```python
from build123d import *

# Parameters (mm, degrees)
BOSS_EXTRUDE1_DEPTH      = 175
BOSS_EXTRUDE1_DEPTH_BACK = 175
SKETCH1_R                = 12.7
SKETCH2_R                = 12.7
BOSS_EXTRUDE2_DEPTH      = 15
BOSS_EXTRUDE3_START      = 15
SKETCH3_R                = 12.7
BOSS_EXTRUDE3_DEPTH      = 15


with BuildPart() as part:
    # Sketch1 → Boss-Extrude1 (new, two sides: drawn at the far end of the back side and taken through both)
    with BuildSketch(Plane(origin=(0, 0, 0), x_dir=(0, 0, -1), z_dir=(1, 0, 0)).offset(-BOSS_EXTRUDE1_DEPTH_BACK)):
        Circle(SKETCH1_R)
    extrude(amount=BOSS_EXTRUDE1_DEPTH + BOSS_EXTRUDE1_DEPTH_BACK)

    # Sketch2 → Boss-Extrude2 (add)
    with BuildSketch(Plane(origin=(175, 0, 0), x_dir=(0, 0, -1), z_dir=(1, 0, 0))):
        Circle(SKETCH2_R)
    extrude(amount=BOSS_EXTRUDE2_DEPTH)

    # Sketch3 → Boss-Extrude3 (add)
    with BuildSketch(Plane.ZY.offset(175).offset(BOSS_EXTRUDE3_START)):
        with Locations(Location((0, 0, 0), (0, 0, 180))):
            Circle(SKETCH3_R)
    extrude(amount=-BOSS_EXTRUDE3_DEPTH)


solid = part.part
```
Can you work these out from the model? Positions are in its coordinate system, mm. Coordinates: 2 decimals unless noted, no trailing zeros. Loops run counter-clockwise (first coordinate to the right, second up) from the corner with the lowest first, then second, coordinate; pieces in that order, holes last. Notation, with made-up numbers: (12, 47) - (54, 47) arc R34 cw to (54, 77) - close; hole circle Ø7 at (-39, 61). An arc over 180 degrees is marked (long way). Use a Markdown table: item, result.
Item 1: I want a section at B-B on y = 8.25. Please give me the cut outline in (x, z).
Numbers:
| item | result |
|---|---|
| outline | (-190, -9.66) - (190, -9.66) - (190, 9.66) - (-190, 9.66) - close |
Item 2: I want a section at A-A on x = -156. Please give me the cut outline in (y, z), and give its area (3 significant figures).
Numbers:
| item | result |
|---|---|
| outline | circle Ø25.4 at (0, 0) |
| area | 507 mm2 |
Item 3: I want a section at C-C on z = 2.75. Please give me the cut outline in (x, y), and give its area (3 significant figures).
Numbers:
| item | result |
|---|---|
| outline | (-190, -12.4) - (190, -12.4) - (190, 12.4) - (-190, 12.4) - close |
| area | 9,420 mm2 |
Item 4: If I drill on probe 1 along Z at (x, y) = (50, 0.25); probe 2 along Z at (x, y) = (-61, 2.75); probe 3 along Y at (x, z) = (85, -4.5), over which ranges is the centre line in solid material (lowest first)? Write a range as from..to.
Numbers:
| item | result |
|---|---|
| probe 1 | z = -12.7..12.7 |
| probe 2 | z = -12.4..12.4 |
| probe 3 | y = -11.88..11.88 |
Item 5: Will these pins go through, and if not, where does the flat tip stop? pin 1 (4 mm diameter, centred on x = 18, y = -6.5, fed in from -Z); pin 2 (5 mm diameter, centred on x = 33, z = -5.5, fed in from +Y); pin 3 (10 mm diameter, centred on x = 120.5, y = -6.5, fed in from -Z).
Numbers:
| item | result |
|---|---|
| pin 1 | stops at z = -11.88 |
| pin 2 | stops at y = 12.34 |
| pin 3 | stops at z = -12.61 |
